from build123d import *

# Parameters (mm, degrees)
SKETCH1_W           = 80
SKETCH1_H           = 60
BOSS_EXTRUDE1_DEPTH = 6
SKETCH2_W           = 5
SKETCH2_H           = 17
BOSS_EXTRUDE2_DEPTH = 11.5
BOSS_EXTRUDE3_DEPTH = 6
BOSS_EXTRUDE4_START = 6
BOSS_EXTRUDE4_DEPTH = 6
BOSS_EXTRUDE5_DEPTH = 2
SKETCH6_W           = 30.556561627
SKETCH6_H           = 19.5
BOSS_EXTRUDE6_DEPTH = 2
FILLET1_R           = 10
FILLET2_R           = 2
BOSS_EXTRUDE7_DEPTH = 5
BOSS_EXTRUDE8_DEPTH = 5
FILLET3_START       = -45
FILLET3_DEPTH       = 90
BOSS_EXTRUDE9_REACH = 101.243
CUT_EXTRUDE1_DEPTH  = 67.535252268


with BuildPart() as part:
    # Sketch1 → Boss-Extrude1 (new body)
    with BuildSketch(Plane(origin=(0, 0, 0), x_dir=(1, 0, 0), z_dir=(0, 1, 0))):
        Rectangle(SKETCH1_W, SKETCH1_H)
    extrude(amount=BOSS_EXTRUDE1_DEPTH)



with BuildPart() as body_2:
    # Sketch2 → Boss-Extrude2 (new body)
    with BuildSketch(Plane(origin=(0, 6, 0), x_dir=(1, 0, 0), z_dir=(0, 1, 0))):
        with BuildLine():
            Line((-45, -13), (-40, -13))
            Line((-40, -13), (-40, 0))
            ThreePointArc((-40, 0), (-43.110841292, -6.265061041), (-45, -13))
        make_face()
        with Locations((-42.5, -21.5)):
            Rectangle(SKETCH2_W, SKETCH2_H)
        with BuildLine():
            Line((40, 0), (40, -13))
            Line((40, -13), (45, -13))
            ThreePointArc((45, -13), (43.110841292, -6.265061041), (40, 0))
        make_face()
        with Locations((42.5, -21.5)):
            Rectangle(SKETCH2_W, SKETCH2_H)
    extrude(amount=BOSS_EXTRUDE2_DEPTH)


with BuildPart() as part_1:
    add(part.part)

    add(body_2.part)  # Boss-Extrude3 merges body 2
    # Sketch3 → Boss-Extrude3 (add)
    with BuildSketch(Plane.XZ.offset(-6)):
        with BuildLine():
            Line((-40, 0), (-40, 30))
            Line((-40, 30), (-45, 30))
            Line((-45, 30), (-45, 13))
            ThreePointArc((-45, 13), (-43.110841292, 6.265061041), (-40, 0))
        make_face()
    extrude(amount=BOSS_EXTRUDE3_DEPTH)

    # Sketch4 → Boss-Extrude4 (add)
    with BuildSketch(Plane.XZ.offset(-6).offset(BOSS_EXTRUDE4_START)):
        with BuildLine():
            Line((40, 30), (40, 0))
            ThreePointArc((40, 0), (43.110841292, 6.265061041), (45, 13))
            Line((45, 13), (45, 30))
            Line((45, 30), (40, 30))
        make_face()
    extrude(amount=-BOSS_EXTRUDE4_DEPTH)

    # Sketch5 → Boss-Extrude5 (add)
    with BuildSketch(Plane(origin=(0, 17.5, 0), x_dir=(1, 0, 0), z_dir=(0, 1, 0))):
        with BuildLine():
            Line((-14.443438373, -30), (-25, -30))
            Line((-25, -30), (-45, -30))
            Line((-45, -30), (-45, -13))
            Line((-45, -13), (-31.955163637, -13))
            ThreePointArc((-31.955163637, -13), (-26.592535057, -14.559489665), (-22.902499246, -18.751557058))
            ThreePointArc((-22.902499246, -18.751557058), (-19.254329924, -24.812974066), (-14.443438373, -30))
        make_face()
        with BuildLine():
            Line((45, -30), (45, -13))
            Line((45, -13), (31.955163637, -13))
            ThreePointArc((31.955163637, -13), (26.592535057, -14.559489665), (22.902499246, -18.751557058))
            ThreePointArc((22.902499246, -18.751557058), (19.254329924, -24.812974066), (14.443438373, -30))
            Line((14.443438373, -30), (25, -30))
            Line((25, -30), (45, -30))
        make_face()
    extrude(amount=BOSS_EXTRUDE5_DEPTH)

    # Sketch6 → Boss-Extrude6 (add)
    with BuildSketch(Plane.XY.offset(30)):
        with Locations((-29.721719186, 9.75)):
            Rectangle(SKETCH6_W, SKETCH6_H)
        with Locations((29.721719186, 9.75)):
            Rectangle(SKETCH6_W, SKETCH6_H)
    extrude(amount=BOSS_EXTRUDE6_DEPTH)

    # Fillet1
    # the kernel refuses this fillet: 10 mm, written as the material it adds along each edge
    with BuildSketch(Plane(origin=(14.443438373, 0, 30), x_dir=(-1, 0, 0), z_dir=(0, 1, 0))) as fillet1_piece_1:
        with BuildLine():
            CenterArc((6, 10), FILLET1_R, 233.130102354, 36.869897646)
            Line((0, 2), (0, 0))
            Line((0, 0), (6, 0))
        make_face()
    extrude(amount=6)
    with BuildSketch(Plane(origin=(-14.443438373, 0, 30), x_dir=(1, 0, 0), z_dir=(0, 1, 0))) as fillet1_piece_2:
        with BuildLine():
            CenterArc((6, -10), FILLET1_R, 90, 36.869897646)
            Line((0, -2), (0, 0))
            Line((0, 0), (6, 0))
        make_face()
    extrude(amount=6)

    # Fillet2
    fillet2_edges = [part_1.edges().sort_by_distance(p)[0] for p in [
        (38.477581818, 19.5, 13),
        (19.254329924, 19.5, 24.812974066),
        (-19.254329924, 19.5, 24.812974066),
        (-26.592535057, 19.5, 14.559489665),
        (26.592535057, 19.5, 14.559489665),
        (-38.477581818, 19.5, 13),
    ]]
    fillet(fillet2_edges, radius=FILLET2_R - 0.0001)  # a hair under: the kernel refuses the full size

    # Sketch7 → Boss-Extrude7 (add)
    with BuildSketch(Plane.XY.offset(32)):
        with BuildLine():
            Line((45, 19.5), (15.184151192, 19.5))
            add(Edge.make_bspline(
                [(15.184151192, 19.5), (14.93580845, 19.5), (14.688907154, 19.481115197), (14.443438373, 19.443462601)],
                knots=[0, 0, 0, 0, 1, 1, 1, 1], degree=3))
            Line((14.443438373, 19.443462601), (14.443438373, 6))
            Line((14.443438373, 6), (14.443438373, 0))
            Line((14.443438373, 0), (45, 0))
            Line((45, 0), (45, 19.5))
        make_face()
    extrude(amount=BOSS_EXTRUDE7_DEPTH)

    # Sketch8 → Boss-Extrude8 (add)
    with BuildSketch(Plane.XY.offset(32)):
        with BuildLine():
            Line((-14.443438373, 6), (-14.443438373, 19.443462601))
            add(Edge.make_bspline(
                [(-14.443438373, 19.443462601), (-14.688907154, 19.481115197), (-14.93580845, 19.5), (-15.184151192, 19.5)],
                knots=[0, 0, 0, 0, 1, 1, 1, 1], degree=3))
            Line((-15.184151192, 19.5), (-45, 19.5))
            Line((-45, 19.5), (-45, 0))
            Line((-45, 0), (-14.443438373, 0))
            Line((-14.443438373, 0), (-14.443438373, 6))
        make_face()
    extrude(amount=BOSS_EXTRUDE8_DEPTH)

    # Fillet3: read off the stored shape, not the designer's step
    # Fillet3 outline → Fillet3 (cut)
    with BuildSketch(Plane.YZ.offset(FILLET3_START)):
        with BuildLine():
            Line((19.5, 37), (9.5, 37))
            ThreePointArc((9.5, 37), (16.571067812, 34.071067812), (19.5, 27))
            Line((19.5, 27), (19.5, 37))
        make_face()
    extrude(amount=FILLET3_DEPTH, mode=Mode.SUBTRACT)

    # Boss-Extrude9: up to this face of the body (flat: up to its plane)
    boss_extrude9_end = Plane(part_1.part.faces().sort_by_distance((-45, 9.370161856, 24.55198813))[0])
    # Sketch9 → Boss-Extrude9 (add, up to the picked face)
    with BuildSketch(Plane(origin=(45, 0, 0), x_dir=(0, 0, -1), z_dir=(1, 0, 0)), mode=Mode.PRIVATE) as boss_extrude9_sk1:
        with BuildLine():
            Line((-37, 0), (-18.411320002, 0))
            ThreePointArc((-18.411320002, 0), (-20.982100343, -5.549822615), (-18.87559935, -11.291956033))
            Line((-18.87559935, -11.291956033), (3.230584985, -29.841247155))
            Line((3.230584985, -29.841247155), (1.302222156, -32.139380484))
            Line((1.302222156, -32.139380484), (-37, 0))
        make_face()
    boss_extrude9_tool1 = split(extrude(boss_extrude9_sk1.sketch, amount=-BOSS_EXTRUDE9_REACH, mode=Mode.PRIVATE), bisect_by=boss_extrude9_end, keep=Keep.BOTH, mode=Mode.PRIVATE)
    add(boss_extrude9_tool1.solids().sort_by(Axis((45, -11.881572, 18.599139), (-1, 0, 0)))[0])

    # Sketch10 → Cut-Extrude1 (cut, through all)
    with BuildSketch(Plane(origin=(0, 0, 0), x_dir=(1, 0, 0), z_dir=(0, 1, 0))):
        with BuildLine():
            Line((-14.443438373, -37), (14.443438373, -37))
            Line((14.443438373, -37), (14.443438373, -32))
            ThreePointArc((14.443438373, -32), (11.605716034, -30.513167019), (8.443438373, -30))
            Line((8.443438373, -30), (-8.443438373, -30))
            ThreePointArc((-8.443438373, -30), (-11.605716034, -30.513167019), (-14.443438373, -32))
            Line((-14.443438373, -32), (-14.443438373, -37))
        make_face()
    extrude(amount=-CUT_EXTRUDE1_DEPTH, mode=Mode.SUBTRACT)


solid = part_1.part
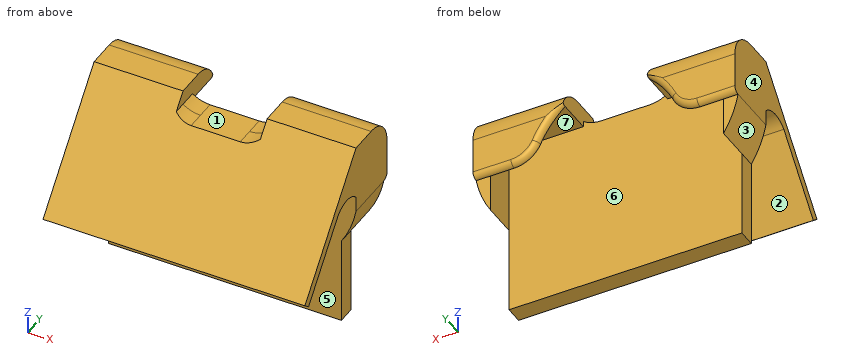
Input: part model. Units: mm. Frame: model coordinates. Face numbers are marked on the shaded views. A direction names the side the tool comes from. Coordinates: 2 decimals unless noted, no trailing zeros. Order: outer loops, then holes, each group sorted by start corner. A loop starts at its lowest first (then second) coordinate and runs counter-clockwise, first axis right, second up. Notation, with made-up numbers: M 3,41.5 L 57,41.5 A13 cw 57,45.5 Z; hole C 28.25,59 d2. An arc over 180 degrees is marked long. Write item = value, one per line. Start each with the question number.
(1) Section A-A on x = -2. Output: boundary loops of the cut face in (y, z).
(2) Pull-direction query (X, two-part tool) for the marked faces 4, 5, 6 and 7; classes: released by +X, released by -X, zero draft, split by the parting line, or undercut.
(3) Section D-D on y = 5. Output: boundary loops of the cut face in (x, z).
(4) Reachability of the marked faces 1, 2 and 3 from +Z, -Z, +X, -X, +Y, -Y: full face, straight path, thin tool, end or side. Return the list, or none.
(5) Section C-C on y = 16.5. Output: boundary loops of the cut face in (x, z).
(6) Line query: line 1 along X through (y, z) = (15.5, 25.5); line 2 along Y through (x, z) = (-17.5, -6); line 3 along Y through (x, z) = (2.5, 11.5). Output: solid intervals per line, ascending. Write a range as [from, to].
(7) Section B-B on z = 1. Output: boundary loops of the cut face in (x, y).
(8) First-contact query: P1, Ø3.5, axis at x = 28.5, y = 10.5, coming from the -Z side; P2, Ø10, axis at x = 22, z = -17, coming from the -Y side; P3, Ø3, axis at x = 18.5, y = -21, coming from the -Z side; P4, Ø24, axis at x = -4, z = -8.5, coming from the -Y side. Flat tips, straight axial feed; report the tip coordinate or a pass-through.
Result set:
q1.outline = M -32.14,-1.3 L -29.84,-3.23 L -11.29,18.88 A7.99 cw 0,18.41 L 0,-30 L 6,-30 L 6,30 L -5.87,30 Z
q2.face_4 = released by -X
q2.face_5 = zero draft
q2.face_6 = undercut
q2.face_7 = undercut
q3.outline = M -45,13 A37.38 ccw -40,0 L -40,-30 L 40,-30 L 40,0 A37.38 ccw 45,13 L 45,37 L 14.44,37 L 14.44,32 A10 cw 8.44,30 L -8.44,30 A10 cw -14.44,32 L -14.44,37 L -45,37 Z
q4.face_1 = +Z, +Y, -Y
q4.face_2 = -Z, +X, -X
q4.face_3 = -Z, -X, +Y
q5.outline = M -45,13 A37.38 ccw -40,0 L -40,30 L -14.44,30 L -14.44,34.14 L -45,34.14 Z; M 14.44,30 L 40,30 L 40,0 A37.38 ccw 45,13 L 45,34.14 L 14.44,34.14 Z
q6.line_1 = [-45, -40], [40, 45]
q6.line_2 = [0, 6]
q6.line_3 = [-21.4, -17.48], [0, 6]
q7.outline = M -45,-30.21 L 45,-30.21 L 45,-26.29 L -45,-26.29 Z; M -40.6,0 L 40.6,0 L 40.6,17.5 L 40,17.5 L 40,6 L -40,6 L -40,17.5 L -40.6,17.5 Z
q8.P1 = 30
q8.P2 = 0
q8.P3 = 5.52
q8.P4 = -32.14
